Build history of the part. All positions in model axes, mm. Face numbers are marked on the shaded views. Round coordinates to 2 decimals unless told otherwise and drop trailing zeros. Order: outer loops, then holes, each group sorted by start corner. A loop starts at its lowest first (then second) coordinate and runs counter-clockwise, first axis right, second up. Notation, with made-up numbers: (19, 69) -> (31, 69) arc R19 cw to (31, 98) -> close; hole circle Ø6 at (77.25, 18.5). An arc over 180 degrees is marked (long way). Answer as a JSON object with one key per item and string values.
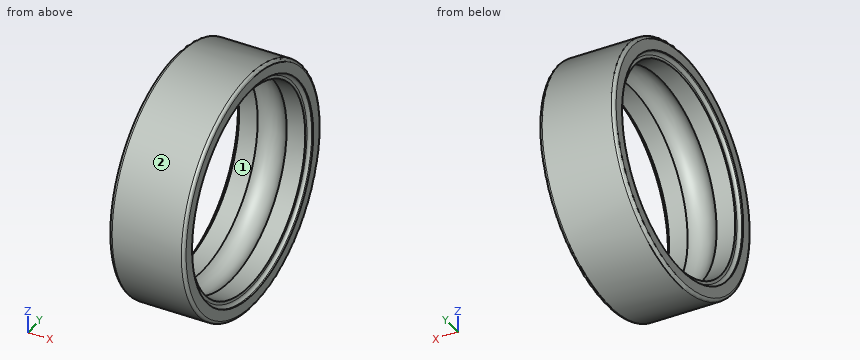
Solid Edge part; units mm, degrees
sketch "Sketch1" plane through (0, 0, 0) normal (0, 0, 1) x (1, 0, 0)
  line L0 (0, 7.8) -> (0, 7.1)
  line L1 (0, 7.1) -> (0.1, 7.1)
  arc A0 (0.1, 7.1) -> (0.3, 6.9) centre (0.1, 6.9) cw
  line L2 (0.3, 6.9) -> (0.3, 6.7)
  line L3 (0.3, 6.7) -> (1.537, 6.7)
  arc A1 (1.537, 6.7) -> (3.463, 6.7) centre (2.5, 6) cw
  line L4 (3.463, 6.7) -> (4.7, 6.7)
  line L5 (4.7, 6.7) -> (4.7, 6.9)
  arc A2 (4.7, 6.9) -> (4.9, 7.1) centre (4.9, 6.9) cw
  line L6 (4.9, 7.1) -> (5, 7.1)
  line L7 (5, 7.1) -> (5, 7.8)
  arc A3 (5, 7.8) -> (4.8, 8) centre (4.8, 7.8) ccw
  line L8 (4.8, 8) -> (0.2, 8)
  arc A4 (0.2, 8) -> (0, 7.8) centre (0.2, 7.8) ccw
revolve "RevolvedProtrusion1" add sketch "Sketch1" angle 360 about axis through (50, 0, 0) along (-1, 0, 0)
properties part number "SKF_628/8-2RS1_or"
1) Pull direction Z, two halves, no side cores. Call the marked faces 1 and 2: pulls with the +Z half, pulls with the -Z half, needs draft (parallel to the pull), parting line crosses it, or undercut.
Checked values:
{"face 1": "undercut", "face 2": "parting line crosses it"}
2) Flat gauge pins, fed straight in: pin 1 Ø2 at (x, z) = (2, 4) entering from +Y; pin 2 Ø1.5 at (x, z) = (3.5, -1) entering from +Y; pin 3 Ø3 at (x, z) = (4.5, 5) entering from -Y. Where does each tip first touch, or does it go through?
Checked values:
{"pin 1": "stops at y = 7.42", "pin 2": "stops at y = 8", "pin 3": "stops at y = -7.19"}
3) Probe L1, parallel to Y at x = 4.4, z = 0; L2, parallel to Z at x = 4, y = -2.75; L3, parallel to Z at x = 0.45, y = 5.25. List the from-to ranges inside material, lowest first. Write a range as from..to.
Checked values:
{"L1": "y = -8..-6.7, 6.7..8", "L2": "z = -7.51..-6.11, 6.11..7.51", "L3": "z = -6.04..-4.16, 4.16..6.04"}
4) Cut at A-A, the plane z = 0. Give the cut face in (x, y).
Checked values:
{"outline": "(0, -7.8) arc R0.2 ccw to (0.2, -8) -> (4.8, -8) arc R0.2 ccw to (5, -7.8) -> (5, -7.1) -> (4.9, -7.1) arc R0.2 cw to (4.7, -6.9) -> (4.7, -6.7) -> (3.46, -6.7) arc R1.19 cw to (1.54, -6.7) -> (0.3, -6.7) -> (0.3, -6.9) arc R0.2 cw to (0.1, -7.1) -> (0, -7.1) -> close; (0, 7.1) -> (0.1, 7.1) arc R0.2 cw to (0.3, 6.9) -> (0.3, 6.7) -> (1.54, 6.7) arc R1.19 cw to (3.46, 6.7) -> (4.7, 6.7) -> (4.7, 6.9) arc R0.2 cw to (4.9, 7.1) -> (5, 7.1) -> (5, 7.8) arc R0.2 ccw to (4.8, 8) -> (0.2, 8) arc R0.2 ccw to (0, 7.8) -> close"}
5) Cut at C-C, the plane x = 4.5. Give the cut face in (y, z), plus the area to 3 significant figures.
Checked values:
{"outline": "circle Ø16 at (0, 0); hole circle Ø13.4 at (0, 0)", "area": "60.0 mm²"}
6) Cut at D-D, the plane x = 2.5. Give the cut face in (y, z).
Checked values:
{"outline": "circle Ø16 at (0, 0); hole circle Ø14.38 at (0, 0)"}
